Autodesk Inventor part; units mm, degrees
ref_plane "YZ Plane" through (0, 0, 0) normal (1, 0, 0) x (0, 1, 0)
ref_plane "XZ Plane" through (0, 0, 0) normal (0, 1, 0) x (-1, 0, 0)
ref_plane "XY Plane" through (0, 0, 0) normal (0, 0, 1) x (1, 0, 0)
sketch "Sketch1" plane through (0, 0, 0) normal (0, 1, 0) x (-1, 0, 0)
  circle A0 centre (0, 0) radius 5.5372 construction
  line L0 (-3.1969, -5.5372) -> (-6.3938, 0)
  line L1 (-6.3938, 0) -> (-3.1969, 5.5372)
  line L2 (-3.1969, 5.5372) -> (3.1969, 5.5372)
  line L3 (3.1969, 5.5372) -> (6.3938, 0)
  line L4 (6.3938, 0) -> (3.1969, -5.5372)
  line L5 (3.1969, -5.5372) -> (-3.1969, -5.5372)
  point P0 (0, -5.5372)
  dimension "d0" = 11.0744
extrude "Extrusion1" add sketch "Sketch1" along normal blind 4.445
sketch "Sketch2" plane through (0, 0, 0) normal (0, -1, 0) x (1, 0, 0)
  circle A0 centre (0, 0) radius 5.08
  circle A1 centre (0, 0) radius 2.794
  dimension "d3" = 10.16
  dimension "d4" = 5.588
extrude "Extrusion2" add sketch "Sketch2" along normal blind 9.525
properties part number "am-2024" material "Brass"
For this review, take the finished solid that the model builds, in its own axes (mm). A direction names the side the tool comes from. Coordinates: 2 decimals unless noted, no trailing zeros. Order: outer loops, then holes, each group sorted by start corner. A loop starts at its lowest first (then second) coordinate and runs counter-clockwise, first axis right, second up. Notation, with made-up numbers: (-25.75, 61) -> (11.25, 61) arc R25 cw to (11.25, 96) -> close; hole circle Ø11 at (62, 77.5). An arc over 180 degrees is marked (long way). Return JSON: item names as keys, results as strings.
1. Machinability: for faces 1 (the cylindrical face through (-0.661, -4.696, -5.037)), 2 (the flat face through (2.2, -9.525, -2.2)), which of the approach directions +Z, -Z, +X, -X, +Y, -Y give a long, thin tool a straight path to every point of the face, cutting with its end or side? Answer none if there is none.
Answer block:
{"face 1": "-Y", "face 2": "+Z, -Z, +X, -X, -Y"}
2. The part is to be moulded in two halves that separate along X. For faces 3 (the flat face through (0, 0, 0)), 4 (the flat face through (0, 2, -5.537)), 5 (the flat face through (-4.818, 2.191, -2.73)), 6 (the cylindrical face through (-2.217, -4.696, 1.7)), say which applies: +X half, -X half, draft (parallel to the pull), parting line (faces both ways), or undercut.
Answer block:
{"face 3": "undercut", "face 4": "draft", "face 5": "-X half", "face 6": "undercut"}
3. For pin 1 Ø3.5 at (x, z) = (2, 0.5) entering from -Y (3 decimals); pin 2 Ø1.5 at (y, z) = (2, -2.5) entering from +X; pin 3 Ø2 at (y, z) = (-5.5, 2.5) entering from -X; pin 4 Ø4 at (x, y) = (-4.5, -3) entering from -Z, all flat-tipped, find the tip position at first contact; note any pin that passes through.
Answer block:
{"pin 1": "y = -9.525", "pin 2": "x = 5.38", "pin 3": "x = -4.85", "pin 4": "z = -4.42"}
4. For line 1 (Z direction, x = 0, y = -2.25); line 2 (Y direction, x = -5.5, z = 0.5) (3 decimals); line 3 (Z direction, x = 0.5, y = -2.5), list the stretches that pass through material, from the lowest coordinate up. Write a range as from..to.
Answer block:
{"line 1": "-5.08..-2.79, 2.79..5.08", "line 2": "0..4.445", "line 3": "-5.06..-2.75, 2.75..5.06"}
5. We need section B-B on x = 0. Write out the cut boundary in (y, z) (3 decimals), and give its area (3 significant figures).
Answer block:
{"outline": "(-9.525, -5.08) -> (0, -5.08) -> (0, -5.537) -> (4.445, -5.537) -> (4.445, 5.537) -> (0, 5.537) -> (0, 5.08) -> (-9.525, 5.08) -> (-9.525, 2.794) -> (0, 2.794) -> (0, -2.794) -> (-9.525, -2.794) -> close", "area": "92.8 mm²"}
6. We need section C-C on z = -3. Write out the cut boundary in (x, y) (3 decimals), and give its area (3 significant figures).
Answer block:
{"outline": "(-4.662, 0) -> (-4.1, 0) -> (-4.1, -9.525) -> (4.1, -9.525) -> (4.1, 0) -> (4.662, 0) -> (4.662, 4.445) -> (-4.662, 4.445) -> close", "area": "120 mm²"}
7. We need section D-D on y = 0.25. Write out the cut boundary in (x, z), and give its area (3 significant figures).
Answer block:
{"outline": "(-6.39, 0) -> (-3.2, -5.54) -> (3.2, -5.54) -> (6.39, 0) -> (3.2, 5.54) -> (-3.2, 5.54) -> close", "area": "106 mm²"}
8. We need section A-A on y = -4. Write out the cut boundary in (x, z).
Answer block:
{"outline": "circle Ø10.16 at (0, 0); hole circle Ø5.59 at (0, 0)"}
